Job drawing, mm, ordinate dimensions from the low corner. One solid piece. A direction names the side the tool comes from. Coordinates: 2 decimals unless noted, no trailing zeros. Order: outer loops, then holes, each group sorted by start corner. A loop starts at its lowest first (then second) coordinate and runs counter-clockwise, first axis right, second up. Notation, with made-up numbers: M 68,-28 L 105,-28 A19 cw 105,-3 Z; hole C 29,43.5 d3. An arc over 180 degrees is marked long. Write item = value, one per line.
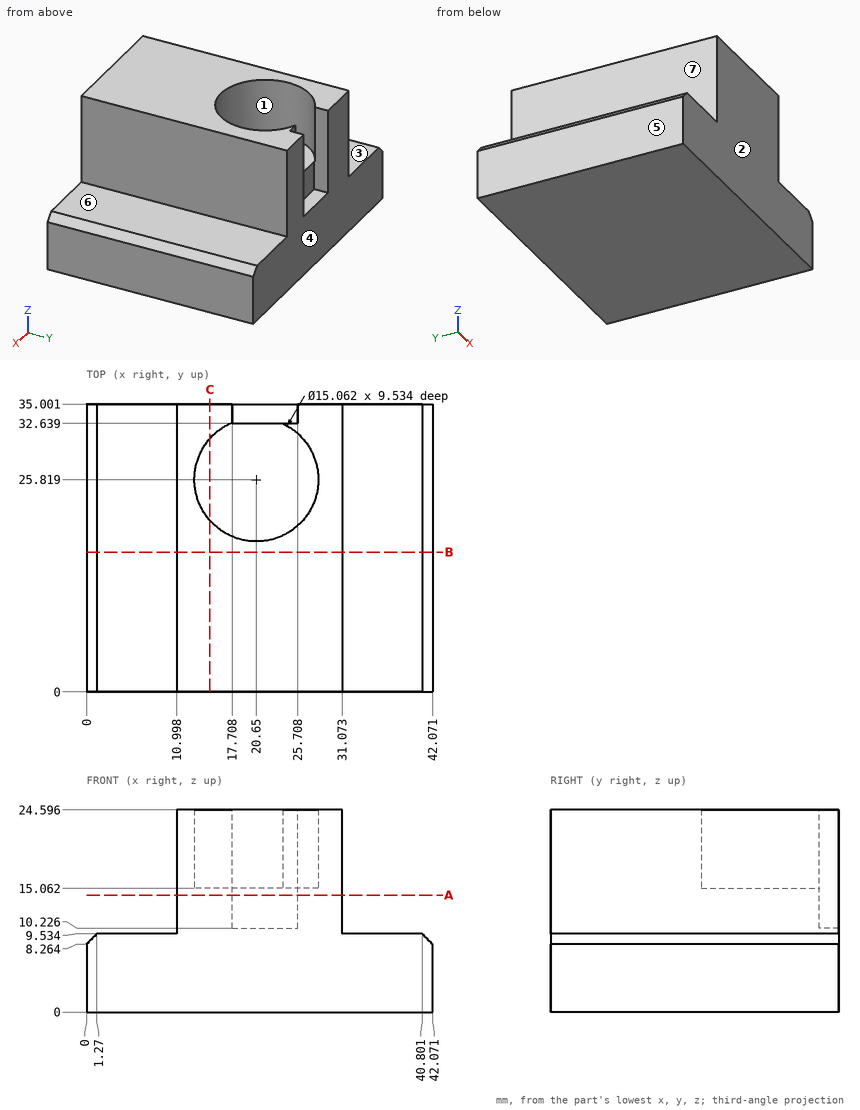
(1) Wall check: line 1 (X direction, y = 26, z = 10.5); line 2 (Z direction, x = 10, y = 8); line 3 (Y direction, x = 25, z = 13.25). Give the ranges that are in metal, low to high. Write a range as from..to.
Evaluation:
line_1 = 11..31.07
line_2 = 0..9.53
line_3 = 0..32.64
(2) Pull direction Y, two halves, no side cores. Call the marked faces 1, 2, 3 and 4: +Y half, -Y half, draft (parallel to the pull), parting line (faces both ways), or undercut.
Evaluation:
face_1 = undercut
face_2 = -Y half
face_3 = draft
face_4 = +Y half
(3) Slice it at C-C, the plane x = 15. Write the cut outline in (y, z) (1 decimal).
Evaluation:
outline = M 0,0 L 35,0 L 35,24.6 L 30.8,24.6 L 30.8,15.1 L 20.8,15.1 L 20.8,24.6 L 0,24.6 Z
(4) Slice it at A-A, the plane z = 14.25. Write the cut outline in (x, y).
Evaluation:
outline = M 11,0 L 31.07,0 L 31.07,35 L 25.71,35 L 25.71,32.64 L 17.71,32.64 L 17.71,35 L 11,35 Z
(5) Slice it at B-B, the plane y = 17. Write the cut outline in (x, z) (1 decimal).
Evaluation:
outline = M 0,0 L 42.1,0 L 42.1,8.3 L 40.8,9.5 L 31.1,9.5 L 31.1,24.6 L 11,24.6 L 11,9.5 L 1.3,9.5 L 0,8.3 Z
(6) Pin check, flat tips, straight feed: pin 1 Ø1.9 at (y, z) = (34.5, 15) entering from -X; pin 2 Ø3 at (y, z) = (31, 21) entering from +X; pin 3 Ø2 at (x, z) = (23.5, 18.5) entering from +Y. Stop position of each tip, or through.
Evaluation:
pin_1 = 11
pin_2 = 31.07
pin_3 = 32.64
(7) Tool access for the marked faces 5, 6 and 7: list every direction of +Z, -Z, +X, -X, +Y, -Y with a clear straight run to the whole face (end or side of a thin tool).
Evaluation:
face_5 = +Z, -Z, -X, +Y, -Y
face_6 = +Z, +X, +Y, -Y
face_7 = +Z, -X, +Y, -Y
